from build123d import *

# Parameters (mm, degrees)
SKETCH1_R           = 35
BOSS_EXTRUDE1_DEPTH = 30
CUT_EXTRUDE1_DEPTH  = 60
CUT_EXTRUDE2_DEPTH  = 60
SKETCH5_R           = 32
CUT_EXTRUDE3_DEPTH  = 26
FILLET3_R           = 2
FILLET4_R           = 2


with BuildPart() as part:
    # Sketch1 → Boss-Extrude1 (new body)
    with BuildSketch(Plane.XY):
        Circle(SKETCH1_R)
    extrude(amount=BOSS_EXTRUDE1_DEPTH)

    # Sketch3 → Cut-Extrude1 (cut)
    with BuildSketch(Plane(origin=(0, 0, 0), x_dir=(-1, 0, 0), z_dir=(0, 0, -1))):
        with BuildLine():
            ThreePointArc((27.75, 0), (24.75, 3), (21.75, 0))
            Line((21.75, 0), (27.75, 0))
        make_face()
        with BuildLine():
            Line((27.75, 0), (21.75, 0))
            ThreePointArc((21.75, 0), (24.75, -3), (27.75, 0))
        make_face()
        with BuildLine():
            ThreePointArc((19.621320344, -15.378679656), (15.378679656, -15.378679656), (15.378679656, -19.621320344))
            Line((15.378679656, -19.621320344), (19.621320344, -15.378679656))
        make_face()
        with BuildLine():
            Line((19.621320344, -15.378679656), (15.378679656, -19.621320344))
            ThreePointArc((15.378679656, -19.621320344), (18.648050297, -20.271638598), (20.5, -17.5))
            ThreePointArc((20.5, -17.5), (20.271638598, -16.351949703), (19.621320344, -15.378679656))
        make_face()
        with BuildLine():
            ThreePointArc((-14.5, -17.5), (-16.351949703, -14.728361402), (-19.621320344, -15.378679656))
            Line((-19.621320344, -15.378679656), (-15.378679656, -19.621320344))
            ThreePointArc((-15.378679656, -19.621320344), (-14.728361402, -18.648050297), (-14.5, -17.5))
        make_face()
        with BuildLine():
            Line((-15.378679656, -19.621320344), (-19.621320344, -15.378679656))
            ThreePointArc((-19.621320344, -15.378679656), (-19.621320344, -19.621320344), (-15.378679656, -19.621320344))
        make_face()
    extrude(amount=-CUT_EXTRUDE1_DEPTH, mode=Mode.SUBTRACT)

    # Sketch3<3> → Cut-Extrude2 (cut)
    with BuildSketch(Plane(origin=(0, 0, 0), x_dir=(-1, 0, 0), z_dir=(0, 0, -1))):
        with BuildLine():
            ThreePointArc((3, -24.75), (2.121320344, -22.628679656), (0, -21.75))
            Line((0, -21.75), (0, -27.75))
            ThreePointArc((0, -27.75), (2.121320344, -26.871320344), (3, -24.75))
        make_face()
        with BuildLine():
            Line((0, -27.75), (0, -21.75))
            ThreePointArc((0, -21.75), (-3, -24.75), (0, -27.75))
        make_face()
        with BuildLine():
            ThreePointArc((-27.75, 0), (-24.75, -3), (-21.75, 0))
            Line((-21.75, 0), (-27.75, 0))
        make_face()
        with BuildLine():
            Line((-27.75, 0), (-21.75, 0))
            ThreePointArc((-21.75, 0), (-24.75, 3), (-27.75, 0))
        make_face()
    extrude(amount=-CUT_EXTRUDE2_DEPTH, mode=Mode.SUBTRACT)

    # Sketch5 → Cut-Extrude3 (cut)
    with BuildSketch(Plane.XY.offset(30)):
        Circle(SKETCH5_R)
    extrude(amount=-CUT_EXTRUDE3_DEPTH, mode=Mode.SUBTRACT)

    # Fillet3
    fillet3_edges = [part.edges().sort_by_distance(p)[0] for p in [
        (-35, 0, 0),
    ]]
    fillet(fillet3_edges, radius=FILLET3_R)

    # Fillet4
    fillet4_edges = [part.edges().sort_by_distance(p)[0] for p in [
        (-32, 0, 4),
    ]]
    fillet(fillet4_edges, radius=FILLET4_R)


solid = part.part
Design review of the part built by this model. Coordinates are the model's own, in mm. A direction names the side the tool comes from. Coordinates: 2 decimals unless noted, no trailing zeros. Loops run counter-clockwise (first coordinate to the right, second up) from the corner with the lowest first, then second, coordinate; pieces in that order, holes last. Notation, with made-up numbers: (-36.5, 59) - (-10.5, 59) arc R23 cw to (-10.5, 72) - close; hole circle Ø1 at (36, -5). An arc over 180 degrees is marked (long way). Use CSV: the item, a comma, the result in double quotes. Start each with the question number.
1. Clearance check with flat-ended pins moving along their axes: pin 1 (7 mm diameter, centred on x = 24.75, y = 0, fed in from -Z); pin 2 (4 mm diameter, centred on y = -18, z = 10, fed in from -X); pin 3 (3 mm diameter, centred on y = -2, z = 21.5, fed in from +X); pin 4 (4 mm diameter, centred on x = 3.5, z = 8.5, fed in from +Y). State where each tip first meets the part, or that it passes through.
2. Add section B-B on z = 13.25. Give the boundary of the cut face in (x, y).
3. To check wall thickness, follow probe 1 along Y at (x, z) = (1, 21.75); probe 2 along Z at (x, y) = (24, -14); probe 3 along X at (y, z) = (-26.5, 14). State the ranges of each line that lie inside material, in increasing order.
4. Add section A-A on y = 0. Give the boundary of the cut face in (x, z).
5. For faces 4 (the cylindrical face through (-6.94, -31.24, 18.17)), 5 (the cylindrical face through (-27.747, -0.132, 1.972)), list the 3-axis set-ups (+Z, -Z, +X, -X, +Y, -Y) from which the entire face can be reached by the end or side of a thin tool; tool diameter is ignored.
6. Mouldability with a two-part tool opening along X and no side actions: class faces 1 (the cylindrical face through (-28, -21, 16)), 2 (the flat face through (15.4, -28.4, 30)), 3 (the flat face through (0, 0, 4)) as released by +X, released by -X, zero draft, split by the parting line, or undercut.
Resolved:
1,pin 1,"z = 0"
1,pin 2,"x = -31.13"
1,pin 3,"x = 35"
1,pin 4,"y = 34.97"
2,outline,"circle Ø70 at (0, 0); hole circle Ø64 at (0, 0)"
3,probe 1,"-34.99 to -31.98, 31.98 to 34.99"
3,probe 2,"0 to 4"
3,probe 3,"-22.86 to -17.94, 17.94 to 22.86"
4,outline,"(-35, 2) arc R2 ccw to (-33, 0) - (-27.75, 0) - (-27.75, 4) - (-30, 4) arc R2 cw to (-32, 6) - (-32, 30) - (-35, 30) - close; (-21.75, 0) - (21.75, 0) - (21.75, 4) - (-21.75, 4) - close; (27.75, 0) - (33, 0) arc R2 ccw to (35, 2) - (35, 30) - (32, 30) - (32, 6) arc R2 cw to (30, 4) - (27.75, 4) - close"
5,face 4,"+Z"
5,face 5,"+Z, -Z"
6,face 1,"split by the parting line"
6,face 2,"zero draft"
6,face 3,"undercut"
